Check sheet for the modelled part. Datum: model origin and axes. Units: mm. A direction names the side the tool comes from. Round coordinates to 2 decimals unless told otherwise and drop trailing zeros. Order: outer loops, then holes, each group sorted by start corner. A loop starts at its lowest first (then second) coordinate and runs counter-clockwise, first axis right, second up. Notation, with made-up numbers: (64.5, 9.25) -> (116.5, 9.25) arc R14 ccw to (116.5, 34.25) -> close; hole circle Ø2 at (-19, 37.25). An arc over 180 degrees is marked (long way). Use CSV: the item, a comma, the result in double quotes.
```python
from build123d import *

# Parameters (mm, degrees)
F0_W     = 96.7861413956
F0_H     = 97.374163568
F1_DEPTH = 50.8
F2_T     = -2.54
F3_R     = 5.08
F4_R     = 5.08


with BuildPart() as f1:
    # F0 (on Top) → F1 (new body)
    with BuildSketch(Plane.XY):
        Rectangle(F0_W, F0_H)
    extrude(amount=F1_DEPTH)

    # F2
    f2_openings = [f1.faces().sort_by_distance(p)[0] for p in [
        (0, 0, 50.8),
    ]]
    offset(amount=F2_T, openings=f2_openings)

    # F3
    f3_edges = [f1.edges().sort_by_distance(p)[0] for p in [
        (-48.393071, -48.687082, 25.4),
        (-48.393071, 48.687082, 25.4),
        (48.393071, 48.687082, 25.4),
        (48.393071, -48.687082, 25.4),
    ]]
    fillet(f3_edges, radius=F3_R)

    # F4
    f4_edges = [f1.edges().sort_by_distance(p)[0] for p in [
        (-45.853071, -46.147082, 26.67),
        (-45.853071, 46.147082, 26.67),
        (45.853071, -46.147082, 26.67),
        (45.853071, 46.147082, 26.67),
    ]]
    fillet(f4_edges, radius=F4_R)


solid = f1.part
```
Q1. Go/stop test with a flat-tipped pin: pin 1 (3 mm diameter, centred on x = 16.5, y = -32, fed in from +Z). Record where the tip stops, or that it passes through.
Result sheet:
pin 1,"stops at z = 2.54"
Q2. Mould release check, pull along X, two halves, no side actions. Record for faces 3 (the face through (48.393, -1, 25)), 4 (the face through (-46.944, -47.159, 25.756)), 5 (the face through (-45.853, -1, 26)), 6 (the face through (-1, 46.147, 26)): pulls with the +X half, pulls with the -X half, needs draft (parallel to the pull), parting line crosses it, or undercut.
Result sheet:
face 3,"pulls with the +X half"
face 4,"pulls with the -X half"
face 5,"undercut"
face 6,"undercut"
Q3. Sectioned sample at A-A, the plane z = 21.5. Enter the section's corners in (x, y), then the cut area to 3 significant figures.
Result sheet:
outline,"(-48.39, -43.61) arc R5.08 ccw to (-43.31, -48.69) -> (43.31, -48.69) arc R5.08 ccw to (48.39, -43.61) -> (48.39, 43.61) arc R5.08 ccw to (43.31, 48.69) -> (-43.31, 48.69) arc R5.08 ccw to (-48.39, 43.61) -> close; hole (-45.85, -41.07) arc R5.08 ccw to (-40.77, -46.15) -> (40.77, -46.15) arc R5.08 ccw to (45.85, -41.07) -> (45.85, 41.07) arc R5.08 ccw to (40.77, 46.15) -> (-40.77, 46.15) arc R5.08 ccw to (-45.85, 41.07) -> close"
area,"961 mm^2"
Q4. Access from +Z, -Z, +X, -X, +Y, -Y to the whole of each face (thin tool, end or side, straight path). Record for faces 1 (the face through (45.853, -1, 26)), 2 (the face through (-46.944, 47.159, 25.756)).
Result sheet:
face 1,"+Z"
face 2,"+Z, -Z, -X, +Y"
Q5. Sectioned sample at B-B, the plane y = -22. Enter the section's corners in (x, z).
Result sheet:
outline,"(-48.39, 0) -> (48.39, 0) -> (48.39, 50.8) -> (45.85, 50.8) -> (45.85, 2.54) -> (-45.85, 2.54) -> (-45.85, 50.8) -> (-48.39, 50.8) -> close"
Q6. Scan lines: L1, parallel to Y at x = -4, z = 33; L2, parallel to X at y = -19, z = 11; L3, parallel to Z at x = -26.5, y = 34. Record each from-to range of solid material in increasing order.
Result sheet:
L1,"y = -48.69 to -46.15, 46.15 to 48.69"
L2,"x = -48.39 to -45.85, 45.85 to 48.39"
L3,"z = 0 to 2.54"
Q7. Sectioned sample at C-C, the plane x = -1.5. Enter the section's corners in (y, z).
Result sheet:
outline,"(-48.69, 0) -> (48.69, 0) -> (48.69, 50.8) -> (46.15, 50.8) -> (46.15, 2.54) -> (-46.15, 2.54) -> (-46.15, 50.8) -> (-48.69, 50.8) -> close"
